Here's the drawing with two shaded views (mm, measured from the low corner). I have some questions. A direction names the side the tool comes from. Round coordinates to 2 decimals unless told otherwise and drop trailing zeros. Write each loop counter-clockwise with the first axis right and the second up, starting at its lowest first coordinate (ties: lowest second). Pieces come first, ordered by that corner, then holes.
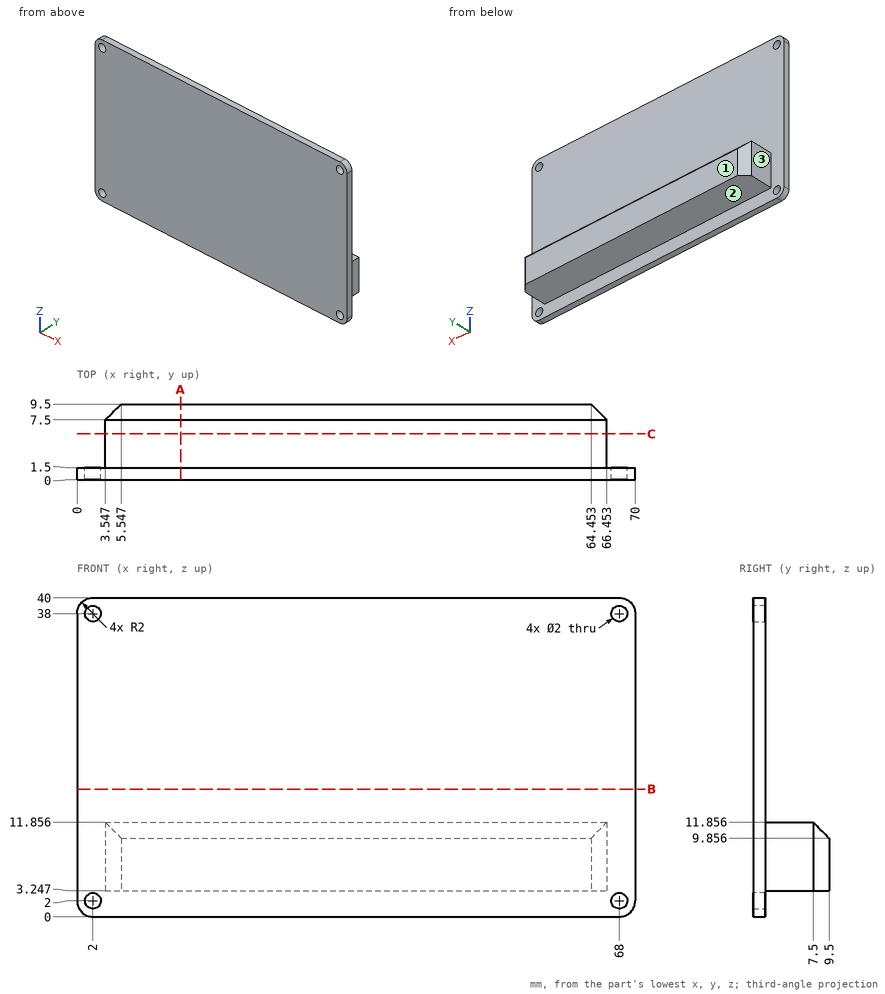
Q1. On a 3-axis mill with a long thin cutter (end or side, diameter ignored), from which of +Z, -Z, +X, -X, +Y, -Y can I reach the whole of each face in a straight line? I mean the marked faces 1, 2 and 3. Say none if no direction works.
Q2. Imagine slicing it at C-C, the plane y = 5.75. Write out the boundary of the cut face in (x, z).
Q3. I'm going to push flat-ended pins straight in: pin 1 Ø10 at (x, z) = (16, 17) entering from -Y; pin 2 Ø1.5 at (x, y) = (8, 8) entering from +Z; pin 3 Ø1.8 at (y, z) = (3.5, 8.5) entering from +X; pin 4 Ø2.5 at (x, z) = (2, 2) entering from +Y. Where does each tip first touch, or does it pass through?
Q4. If I drill on L1, parallel to Z at x = 68, y = 0.8; L2, parallel to X at y = 0.6, z = 38; L3, parallel to Y at x = 37, z = 28.5, over which ranges is the centre line in solid material (lowest first)?
Q5. Imagine slicing it at A-A, the plane x = 13. Write out the boundary of the cut face in (y, z), then the cut area to 3 significant figures.
Q6. Imagine slicing it at B-B, the plane z = 16. Write out the boundary of the cut face in (x, y).
Results found:
1. face 1: +Z, -Z, +X, -X, +Y
1. face 2: -Z, +X, -X, +Y
1. face 3: +Z, -Z, -X, +Y
2. outline: (3.55, 3.25) - (66.45, 3.25) - (66.45, 11.86) - (3.55, 11.86) - close
3. pin 1: stops at y = 0
3. pin 2: stops at z = 11.86
3. pin 3: stops at x = 66.45
3. pin 4: stops at y = 1.5
4. L1: z = 0 to 1, 3 to 37, 39 to 40
4. L2: x = 0 to 1, 3 to 67, 69 to 70
4. L3: y = 0 to 1.5
5. outline: (0, 0) - (1.5, 0) - (1.5, 3.25) - (9.5, 3.25) - (9.5, 9.86) - (7.5, 11.86) - (1.5, 11.86) - (1.5, 40) - (0, 40) - close
5. area: 127 mm2
6. outline: (0, 0) - (70, 0) - (70, 1.5) - (0, 1.5) - close
